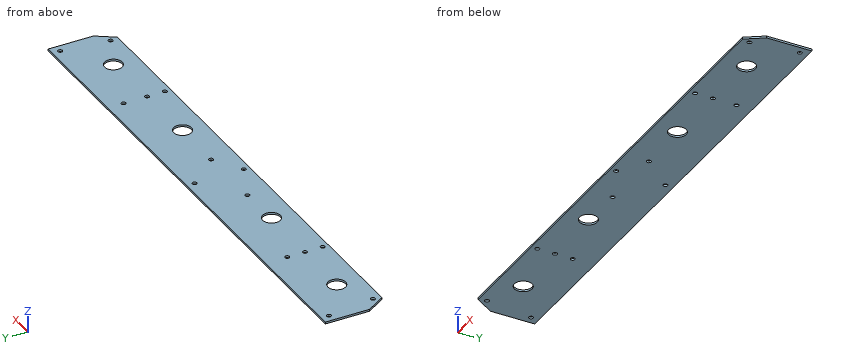
Autodesk Inventor part; units mm, degrees
ref_plane "YZ Plane" through (0, 0, 0) normal (1, 0, 0) x (0, 1, 0)
ref_plane "XZ Plane" through (0, 0, 0) normal (0, 1, 0) x (-1, 0, 0)
ref_plane "XY Plane" through (0, 0, 0) normal (0, 0, 1) x (1, 0, 0)
sketch "Sketch1" plane through (0, 0, 0) normal (0, 0, 1) x (1, 0, 0)
  line L0 (0, 0) -> (850.9, 0)
  line L1 (850.9, 0) -> (850.9, 76.2)
  line L2 (850.9, 76.2) -> (0, 76.2)
  line L3 (0, 76.2) -> (0, 0)
  dimension "d0" = 850.9
  dimension "d1" = 76.2
extrude "Extrusion1" add sketch "Sketch1" along normal blind 3.175
sketch "Sketch4" plane through (0, 0, 3.175) normal (0, 0, 1) x (1, 0, 0)
  line L0 (0, 0) -> (0, 38.1)
  line L1 (0, 76.2) -> (0, 0)
  line L2 (0, 0) -> (25.4, 0)
  line L3 (0, 0) -> (850.9, 0)
  line L4 (25.4, 0) -> (0, 38.1)
  line L5 (850.9, 0) -> (825.5, 0)
  line L6 (850.9, 0) -> (850.9, 38.1)
  line L7 (850.9, 0) -> (850.9, 76.2)
  line L8 (850.9, 38.1) -> (825.5, 0)
  line L9 (0, 38.1) -> (0, 36.5125)
  circle A0 centre (292.9509, 36.5125) radius 14.2875
  circle A1 centre (557.9491, 36.5125) radius 14.2875
  circle A2 centre (757.9743, 39.6875) radius 14.2875
  circle A3 centre (92.9257, 39.6875) radius 14.2875
  dimension "d24" = 38.1
  dimension "d26" = 25.4
  dimension "d27" = 38.1
  dimension "d33" = 28.575
  dimension "d34" = 28.575
  dimension "d38" = 28.575
  dimension "d39" = 28.575
extrude "Extrusion3" cut sketch "Sketch4" against normal blind 3.175
sketch "Sketch5" plane through (0, 0, 3.175) normal (0, 0, 1) x (1, 0, 0)
  line L0 (850.9, 76.2) -> (0, 76.2)
  line L1 (0, 76.2) -> (425.45, 76.2)
  circle A0 centre (425.45, 66.675) radius 3.5687
  circle A1 centre (425.45, 9.525) radius 3.5687
  line L2 (25.4, 0) -> (825.5, 0)
  line L3 (0, 76.2) -> (190.5, 76.2)
  circle A2 centre (190.5, 66.675) radius 3.5687
  circle A3 centre (190.5, 9.525) radius 3.5687
  circle A4 centre (190.5, 38.1) radius 3.5687
  line L4 (850.9, 38.1) -> (850.9, 76.2)
  line L5 (850.9, 76.2) -> (660.4, 76.2)
  circle A5 centre (660.4, 66.675) radius 3.5687
  circle A6 centre (660.4, 9.525) radius 3.5687
  circle A7 centre (660.4, 38.1) radius 3.5687
  circle A8 centre (838.2, 63.5) radius 3.5687
  circle A9 centre (12.7, 63.5) radius 3.5687
  line L6 (0, 76.2) -> (0, 38.1)
  circle A10 centre (34.925, 12.7) radius 3.5687
  circle A11 centre (815.975, 12.7) radius 3.5687
  point P0 (0, 0)
  dimension "d42" = 425.45
  dimension "d43" = 7.1374
  dimension "d44" = 9.525
  dimension "d45" = 7.1374
  dimension "d46" = 9.525
  dimension "d47" = 190.5
  dimension "d48" = 7.1374
  dimension "d49" = 9.525
  dimension "d50" = 7.1374
  dimension "d51" = 9.525
  dimension "d52" = 7.1374
  dimension "d53" = 38.1
  dimension "d54" = 190.5
  dimension "d55" = 7.1374
  dimension "d56" = 9.525
  dimension "d57" = 7.1374
  dimension "d58" = 9.525
  dimension "d59" = 7.1374
  dimension "d60" = 38.1
  dimension "d61" = 7.1374
  dimension "d62" = 12.7
  dimension "d63" = 12.7
  dimension "d64" = 7.1374
  dimension "d65" = 12.7
  dimension "d66" = 12.7
  dimension "d67" = 7.1374
  dimension "d69" = 12.7
  dimension "d70" = 9.525
  dimension "d71" = 7.1374
  dimension "d72" = 12.7
  dimension "d73" = 9.525
extrude "Extrusion4" cut sketch "Sketch5" against normal blind 3.175
sketch "Sketch6" plane through (0, 0, 3.175) normal (0, 0, 1) x (1, 0, 0)
  circle A0 centre (361.95, 38.1) radius 3.5687
  circle A1 centre (469.9, 38.1) radius 3.5687
  line L0 (850.9, 76.2) -> (0, 76.2)
  circle A2 centre (292.9509, 36.5125) radius 14.2875
  line L1 (0, 76.2) -> (0, 38.1)
  line L2 (850.9, 38.1) -> (850.9, 76.2)
  point P0 (0, 0)
  dimension "d76" = 7.1374
  dimension "d77" = 7.1374
  dimension "d78" = 38.1
  dimension "d79" = 38.1
  dimension "d82" = 381
  dimension "d83" = 361.95
extrude "Extrusion6" cut sketch "Sketch6" against normal blind 25.4 contours A0 | A1
sketch "Sketch7" plane through (0, 76.2, 0) normal (0, 1, 0) x (1, 0, 0)
  line L0 (850.9, 0) -> (0, 0)
  line L1 (0, 0) -> (0, -3.175)
  line L2 (850.9, -3.175) -> (0, -3.175)
  line L3 (850.9, 0) -> (850.9, -3.175)
extrude "Extrusion7" add sketch "Sketch7" along normal blind 25.4
sketch "Sketch8" plane through (0, 0, 3.175) normal (0, 0, 1) x (1, 0, 0)
  circle A0 centre (12.7, 63.5) radius 3.5687
  circle A1 centre (838.2, 63.5) radius 3.5687
  circle A2 centre (425.45, 66.675) radius 3.5687
  point P0 (0, 0)
extrude "Extrusion9" add sketch "Sketch8" against normal blind 3.175
sketch "Sketch9" plane through (0, 0, 3.175) normal (0, 0, 1) x (1, 0, 0)
  circle A0 centre (12.7, 88.9) radius 3.5687
  line L0 (0, 101.6) -> (850.9, 101.6)
  line L1 (0, 38.1) -> (0, 101.6)
  circle A1 centre (838.2, 88.9) radius 3.5687
  line L2 (850.9, 38.1) -> (850.9, 101.6)
  circle A2 centre (425.45, 88.9) radius 3.5687
  point P0 (0, 0)
  dimension "d95" = 7.1374
  dimension "d96" = 12.7
  dimension "d97" = 12.7
  dimension "d98" = 7.1374
  dimension "d99" = 12.7
  dimension "d100" = 12.7
  dimension "d101" = 7.1374
extrude "Extrusion10" cut sketch "Sketch9" against normal blind 3.175
sketch "Sketch10" plane through (0, 0, 3.175) normal (0, 0, 1) x (1, 0, 0)
  line L0 (0, 38.1) -> (0, 101.6)
  line L1 (0, 101.6) -> (12.7, 101.6)
  line L2 (0, 101.6) -> (850.9, 101.6)
  line L3 (12.7, 101.6) -> (12.7, 19.05)
  line L4 (0, 38.1) -> (25.4, 0)
  line L5 (850.9, 101.6) -> (838.2, 101.6)
  line L6 (838.2, 101.6) -> (838.2, 19.05)
  line L7 (825.5, 0) -> (850.9, 38.1)
  line L8 (838.2, 19.05) -> (850.9, 38.1)
  line L9 (850.9, 38.1) -> (850.9, 101.6)
  line L10 (850.9, 101.6) -> (850.9, 38.1)
  line L11 (12.7, 19.05) -> (0, 38.1)
  line L12 (0, 101.6) -> (0, 38.1)
  point P0 (0, 0)
  dimension "d104" = 12.7
  dimension "d105" = 12.7
extrude "Extrusion11" cut sketch "Sketch10" against normal blind 25.4
sketch "Sketch11" plane through (0, 0, 3.175) normal (0, 0, 1) x (1, 0, 0)
  arc A0 (12.7, 85.3313) -> (12.7, 92.4687) centre (12.7, 88.9) ccw
  line L0 (12.7, 92.4687) -> (12.7, 85.3313)
  arc A1 (838.2, 92.4687) -> (838.2, 85.3313) centre (838.2, 88.9) ccw
  line L1 (838.2, 92.4687) -> (838.2, 85.3313)
  point P0 (0, 0)
extrude "Extrusion12" add sketch "Sketch11" against normal blind 3.175
sketch "Sketch12" plane through (0, 0, 3.175) normal (0, 0, 1) x (1, 0, 0)
  line L0 (25.4, 0) -> (825.5, 0)
  line L1 (25.4, 0) -> (31.75, 0)
  line L2 (31.75, 0) -> (12.7, 30.4376)
  line L3 (12.7, 19.05) -> (12.7, 101.6)
  line L4 (12.7, 30.4376) -> (12.7, 19.05)
  line L5 (25.4, 0) -> (12.7, 19.05)
  line L6 (12.7, 19.05) -> (25.4, 0)
  line L7 (25.4, 0) -> (31.75, 0)
  line L8 (25.4, 0) -> (12.7, 19.05)
  line L9 (838.2, 19.05) -> (825.5, 0)
  line L10 (825.5, 0) -> (819.15, 0)
  line L11 (819.15, 0) -> (838.2, 28.575)
  line L12 (838.2, 101.6) -> (838.2, 19.05)
  line L13 (838.2, 28.575) -> (838.2, 19.05)
  line L14 (838.2, 19.05) -> (825.5, 0)
  point P0 (0, 0)
  dimension "d111" = 6.35
  dimension "d113" = 6.35
extrude "Extrusion13" cut sketch "Sketch12" against normal blind 3.175
sketch "Sketch13" plane through (0, 0, 3.175) normal (0, 0, 1) x (1, 0, 0)
  circle A0 centre (25.4, 88.9) radius 3.5687
  line L0 (12.7, 101.6) -> (838.2, 101.6)
  line L1 (12.7, 101.6) -> (12.7, 30.4376)
  circle A1 centre (825.5, 88.9) radius 3.5687
  line L2 (838.2, 101.6) -> (838.2, 28.575)
  point P0 (0, 0)
  dimension "d116" = 7.1374
  dimension "d117" = 12.7
  dimension "d118" = 12.7
  dimension "d119" = 7.1374
  dimension "d120" = 12.7
  dimension "d121" = 12.7
extrude "Extrusion14" cut sketch "Sketch13" against normal blind 3.175
sketch "Sketch14" plane through (0, 0, 3.175) normal (0, 0, 1) x (1, 0, 0)
  circle A0 centre (660.4, 66.675) radius 3.5687
  circle A1 centre (660.4, 38.1) radius 3.5687
  point P0 (0, 0)
  dimension "d124" = 28.575
extrude "Extrusion15" add sketch "Sketch14" against normal blind 3.175 contours A0
sketch "Sketch15" plane through (0, 0, 3.175) normal (0, 0, 1) x (1, 0, 0)
  circle A0 centre (660.4, 38.1) radius 3.5687
  circle A1 centre (660.4, 76.2) radius 3.5687
  point P0 (0, 0)
  dimension "d127" = 7.1374
  dimension "d128" = 38.1
extrude "Extrusion16" cut sketch "Sketch15" against normal blind 3.175 contours A1
properties part number "OutsidePlate2" material "Aluminum 6061"
Can you work these out from the model? Positions are in its coordinate system, mm. Coordinates: 2 decimals unless noted, no trailing zeros. Write each loop counter-clockwise with the first axis right and the second up, starting at its lowest first coordinate (ties: lowest second). Pieces come first, ordered by that corner, then holes. Notation, with made-up numbers: (19.25, -27.5) - (23.25, -27.5) arc R35 ccw to (23.25, 9.5) - close; hole circle Ø3 at (2.5, 21.25). An arc over 180 degrees is marked (long way). Return JSON: item names as keys, results as strings. Group by question number.
Item 1: If we section it at A-A (x = 95): Write out the boundary of the cut face in (y, z) (3 decimals).
Item 2: If we section it at B-B (z = 1.8): Count the separate pieces of the cut face and the enclosed holes in it, then the cut area to 3 significant figures.
Item 3: I'm going to push a flat-ended pin straight in: pin 1 Ø5.5 at (x, y) = (425.45, 88.9) entering from -Z. Where does the tip first touch, or does it pass through?
Item 4: Please list where these lines run through material, in increasing order: probe 1 along Y at (x, z) = (660.4, 2.25); probe 2 along X at (y, z) = (27, 2.25); probe 3 along X at (y, z) = (34, 2.4).
Return value:
{
 "1": {"outline": "(0, 0) - (25.551, 0) - (25.551, 3.175) - (0, 3.175) - close; (53.824, 0) - (101.6, 0) - (101.6, 3.175) - (53.824, 3.175) - close"},
 "2": {"separate pieces": "1", "enclosed holes": "18", "area": "80,200 mm^2"},
 "3": {"pin 1": "passes through"},
 "4": {"probe 1": "y = 0 to 5.96, 13.09 to 34.53, 41.67 to 72.63, 79.77 to 101.6", "probe 2": "x = 14.85 to 86.36, 99.5 to 282.29, 303.61 to 547.29, 568.61 to 751.4, 764.54 to 837.15", "probe 3": "x = 12.7 to 79.82, 106.03 to 278.89, 307.02 to 543.88, 572.01 to 744.87, 771.08 to 838.2"}
}
